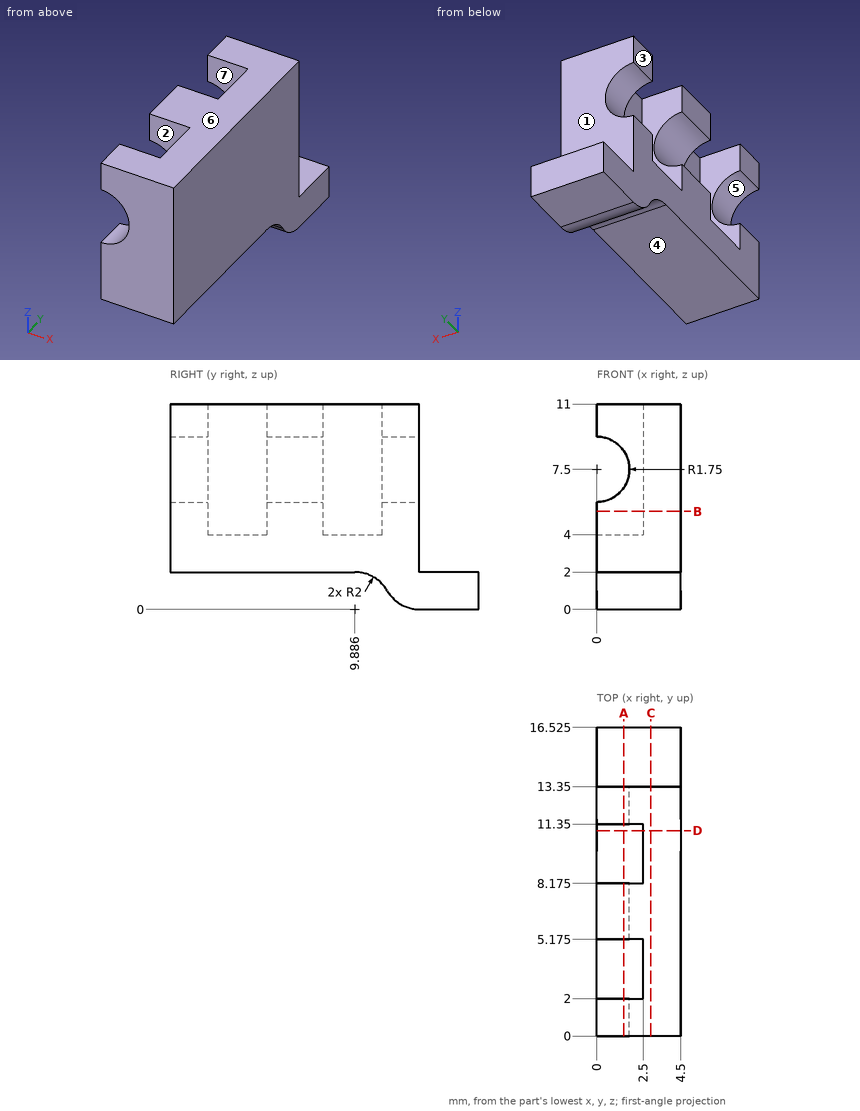
Verification items for this drawing (mm, ordinates from the low corner). A direction names the side the tool comes from. Round coordinates to 2 decimals unless told otherwise and drop trailing zeros. Order: outer loops, then holes, each group sorted by start corner. A loop starts at its lowest first (then second) coordinate and runs counter-clockwise, first axis right, second up.
1) Cross-section at C-C, the plane x = 2.9. Record the cut outline in (y, z) (3 decimals), plus the area to 3 significant figures.
Geometry says:
outline: (0, 2) - (9.886, 2) arc R2 cw to (11.618, 1) arc R2 ccw to (13.35, 0) - (16.525, 0) - (16.525, 2) - (13.35, 2) - (13.35, 11) - (0, 11) - close
area: 130 mm2
2) Cross-section at D-D, the plane y = 11. Record the cut outline in (x, z), plus the area to 3 significant figures.
Geometry says:
outline: (0, 1.66) - (4.5, 1.66) - (4.5, 11) - (2.5, 11) - (2.5, 4) - (0, 4) - close
area: 24.5 mm2
3) Draft check along Z on the marked faces 5, 6 and 7. Enter one of: +Z half, -Z half, draft (parallel to the pull), parting line (faces both ways), or undercut.
Geometry says:
face 5: undercut
face 6: +Z half
face 7: draft
4) Material ranges on line 1 (Y direction, x = 2.45, z = 5.5) (3 decimals); line 2 (Y direction, x = 2.6, z = 9.75); line 3 (Z direction, x = 1.05, y = 4.5), recorded low to high.
Geometry says:
line 1: y = 0 to 2, 5.175 to 8.175, 11.35 to 13.35
line 2: y = 0 to 13.35
line 3: z = 2 to 4
5) Depth check by flat-ended pin: pin 1 (0.8 mm diameter, centred on x = 1, z = 8, fed in from -Y); pin 2 (1.2 mm diameter, centred on x = 0.5, z = 6, fed in from +Y); pin 3 (0.8 mm diameter, centred on x = 1, y = 3.5, fed in from +Z); pin 4 (2.5 mm diameter, centred on x = 3, y = 15.5, fed in from +Z). Enter the tip coordinate at first touch or a pass-through.
Geometry says:
pin 1: passes through
pin 2: stops at y = 13.35
pin 3: stops at z = 4
pin 4: stops at z = 2
6) Cross-section at A-A, the plane x = 1.45. Give the number of separate pieces and of enclosed holes in the cut face, plus the area to 3 significant figures.
Geometry says:
separate pieces: 4
enclosed holes: 0
area: 71.8 mm2
7) Tool access check on the marked faces 1, 2, 3 and 4. Record the directions out of +Z, -Z, +X, -X, +Y, -Y that give a thin tool (end or side, any length) a straight path to the whole face; none if there is none.
Geometry says:
face 1: +Z, +X, -X, +Y
face 2: +Z, -X
face 3: +Z, -Z, -X, +Y, -Y
face 4: -Z, +X, -X, -Y
8) Cross-section at B-B, the plane z = 5.25. Record the cut outline in (x, y) (3 decimals).
Geometry says:
outline: (0, 0) - (4.5, 0) - (4.5, 13.35) - (0, 13.35) - (0, 11.35) - (2.5, 11.35) - (2.5, 8.175) - (0, 8.175) - (0, 5.175) - (2.5, 5.175) - (2.5, 2) - (0, 2) - close
